```python
from build123d import *

# Parameters (mm, degrees)
SKETCH_1_W      = 36
SKETCH_1_H      = 70
SKETCH_1_R      = 1.25
SKETCH_1_W_2    = 12
SKETCH_1_H_2    = 46
EXTRUDE_1_DEPTH = 2.4
FILLET_1_R      = 3


with BuildPart() as part:
    # 草图1 → 凸台-拉伸1 (new body)
    with BuildSketch(Plane(origin=(0, 0, 0), x_dir=(1, 0, 0), z_dir=(0, 1, 0))):
        Rectangle(SKETCH_1_W, SKETCH_1_H)
        with Locations(Location((-9.4, 27.75, 0), (0, 0, 270))):
            Circle(SKETCH_1_R, mode=Mode.SUBTRACT)
        with Locations(Location((9.4, 27.75, 0), (0, 0, 90))):
            Circle(SKETCH_1_R, mode=Mode.SUBTRACT)
        with Locations(Location((9.4, -27.75, 0), (0, 0, 270))):
            Circle(SKETCH_1_R, mode=Mode.SUBTRACT)
        with Locations(Location((-9.4, -27.75, 0), (0, 0, 90))):
            Circle(SKETCH_1_R, mode=Mode.SUBTRACT)
        with Locations(Location((-15, 31.5, 0), (0, 0, 270))):
            Circle(SKETCH_1_R, mode=Mode.SUBTRACT)
        with Locations(Location((15, 31.5, 0), (0, 0, 90))):
            Circle(SKETCH_1_R, mode=Mode.SUBTRACT)
        with Locations(Location((-15, -31.5, 0), (0, 0, 90))):
            Circle(SKETCH_1_R, mode=Mode.SUBTRACT)
        with Locations(Location((15, -31.5, 0), (0, 0, 270))):
            Circle(SKETCH_1_R, mode=Mode.SUBTRACT)
        Rectangle(SKETCH_1_W_2, SKETCH_1_H_2, mode=Mode.SUBTRACT)
    extrude(amount=EXTRUDE_1_DEPTH)

    # 圆角1
    fillet_1_edges = [part.edges().sort_by_distance(p)[0] for p in [
        (-6, 1.2, 23),
        (6, 1.2, 23),
        (6, 1.2, -23),
        (-6, 1.2, -23),
        (18, 1.2, 35),
        (-18, 1.2, 35),
        (-18, 1.2, -35),
        (18, 1.2, -35),
    ]]
    fillet(fillet_1_edges, radius=FILLET_1_R)


solid = part.part
```
The model under review builds one solid part; all positions refer to its coordinate system, in mm. A direction names the side the tool comes from. Round coordinates to 2 decimals unless told otherwise and drop trailing zeros. Order: outer loops, then holes, each group sorted by start corner. A loop starts at its lowest first (then second) coordinate and runs counter-clockwise, first axis right, second up. Notation, with made-up numbers: (-38, 17) -> (-32, 17) arc R14 cw to (-32, 35) -> close; hole circle Ø7 at (36.25, 26.5). An arc over 180 degrees is marked (long way). One line per item, written item: value. Start each with the question number.
Q1. Take a section at D-D (x = 1). Write out the cut boundary in (y, z), and give its area (3 significant figures).
Q2. Machinability: for faces 1 (the face through (-8, 2.4, 0)), 2 (the face through (0, 1, -23)), which of the approach directions +Z, -Z, +X, -X, +Y, -Y give a long, thin tool a straight path to every point of the face, cutting with its end or side? Answer none if there is none.
Q3. Mouldability with a two-part tool opening along X and no side actions: class faces 3 (the face through (-17.14, 1.22, -34.1)), 4 (the face through (0, 1, 35)), 5 (the face through (9.879, 1.183, -28.905)) as released by +X, released by -X, zero draft, split by the parting line, or undercut.
Q4. Clearance check with a flat-ended pin moving along its axis: pin 1 Ø2 at (x, z) = (-9.4, 27.75) entering from -Y. State where the tip first meets the part, or that it passes through.
Q5. Take a section at A-A (x = 9.4). Write out the cut boundary in (y, z), and give its area (3 significant figures).
Q6. Wall thickness on line 1 (X direction, y = 1.4, z = 27.75); line 2 (X direction, y = 0.9, z = 4.5); line 3 (Z direction, x = 2.5, y = 0.55): over which ranges is each line inside the solid? List them lowest first.
Q7. Take a section at B-B (y = 1.2). Count the separate pieces of the cut face and the enclosed holes in it, and give its area (3 significant figures).
Q8. Take a section at C-C (z = -12). Write out the cut boundary in (x, y).
Reported:
1. outline: (0, -35) -> (2.4, -35) -> (2.4, -23) -> (0, -23) -> close; (0, 23) -> (2.4, 23) -> (2.4, 35) -> (0, 35) -> close
1. area: 57.6 mm2
2. face 1: +Z, -Z, +X, -X, +Y
2. face 2: +Y, -Y
3. face 3: released by -X
3. face 4: zero draft
3. face 5: undercut
4. pin 1: passes through
5. outline: (0, -35) -> (2.4, -35) -> (2.4, -29) -> (0, -29) -> close; (0, -26.5) -> (2.4, -26.5) -> (2.4, 26.5) -> (0, 26.5) -> close; (0, 29) -> (2.4, 29) -> (2.4, 35) -> (0, 35) -> close
5. area: 156 mm2
6. line 1: x = -18 to -10.65, -8.15 to 8.15, 10.65 to 18
6. line 2: x = -18 to -6, 6 to 18
6. line 3: z = -35 to -23, 23 to 35
7. separate pieces: 1
7. enclosed holes: 9
7. area: 1,930 mm2
8. outline: (-18, 0) -> (-6, 0) -> (-6, 2.4) -> (-18, 2.4) -> close; (6, 0) -> (18, 0) -> (18, 2.4) -> (6, 2.4) -> close
